Autodesk Inventor part; units mm, degrees
ref_plane "YZ Plane" through (0, 0, 0) normal (1, 0, 0) x (0, 1, 0)
ref_plane "XZ Plane" through (0, 0, 0) normal (0, 1, 0) x (-1, 0, 0)
ref_plane "XY Plane" through (0, 0, 0) normal (0, 0, 1) x (1, 0, 0)
sketch "Sketch1" plane through (0, 0, 0) normal (0, 1, 0) x (-1, 0, 0)
  line L0 (-7.5, 15) -> (7.5, 15)
  line L1 (7.5, 15) -> (7.5, -15)
  line L2 (7.5, -15) -> (-7.5, -15)
  line L3 (-7.5, -15) -> (-7.5, 15)
  line L4 (-7.5, 15) -> (7.5, -15) construction
  line L5 (7.5, 15) -> (-7.5, -15) construction
  point P0 (0, 0)
  dimension "d0" = 15
  dimension "d1" = 30
extrude "Extrusion1" add sketch "Sketch1" along normal blind 4
chamfer "Chamfer1" distance 2.5 distance2 1 1 edges at (7.5, 2, -15) measured on face at (7.5, 1.3333, 5)
chamfer "Chamfer2" distance 1 distance2 2.5 1 edges at (-7.5, 2, -15) measured on face at (1.8333, 2.6667, -15)
sketch "Sketch3" plane through (0, 0, 0) normal (0, -1, 0) x (1, 0, 0)
  line L0 (0, 0) -> (4, 0)
  line L1 (0, 0) -> (-4, 0)
  dimension "d14" = 4
  dimension "d15" = 4
hole "Hole1" at (4, 0, 0) at (-4, 0, 0) direction (0, 1, 0) diameter 2.1565 end through all
sketch "Sketch4" plane through (0, 0, 0) normal (0, -1, 0) x (1, 0, 0)
  line L0 (7.5, 15) -> (7.5, -12.5)
  line L1 (7.5, -12.5) -> (7.5, -7.5)
  line L2 (7.5, -7.5) -> (2.5, -7.5)
  line L3 (2.5, -7.5) -> (2.5, -5.5)
  line L4 (2.5, -5.5) -> (-2.5, -5.5)
  line L5 (-2.5, -5.5) -> (-2.5, -7.5)
  line L6 (-2.5, -7.5) -> (-7.5679, -7.5)
  line L7 (-7.5679, -7.5) -> (-7.5679, -12.5)
  line L8 (6.5, -15) -> (-6.5, -15)
  line L9 (-7.5679, -12.5) -> (-6.5, -15)
  line L10 (7.5, -12.5) -> (6.5, -15)
  line L11 (-6.5, -15) -> (6.5, -15)
  line L12 (6.5, -15) -> (7.5, -12.5)
  point P0 (0, 0)
  dimension "d23" = 5
  dimension "d24" = 5
  dimension "d25" = 2
  dimension "d26" = 5
split body "Split1" sketch "Sketch4" result one side removed curves L2 L3 L4 L5 L6 L7 L9 L11 L12 L1 removed pieces at (1.1663, 0.5, 10.3182)
sketch "Sketch5" plane through (-7.5, 0, -12.5) normal (-1, 0, 0) x (0, 0, 1)
  line L0 (0, 0) -> (0, 4)
  line L1 (-2.5, 4) -> (-2.5, 0)
  line L2 (0, 0) -> (-2.5, 0)
  line L3 (-2.5, 0) -> (-2.5, 4)
  line L4 (-2.5, 4) -> (0, 4)
  line L5 (0, 4) -> (0, 0)
  point P0 (12.5, 0)
extrude "Extrusion3" cut sketch "Sketch5" against normal blind 2
sketch "Sketch6" plane through (7.5, 0, -12.5) normal (1, 0, 0) x (0, 0, -1)
  line L0 (0, 4) -> (0, 0)
  line L1 (2.5, 0) -> (2.5, 4)
  line L2 (0, 4) -> (2.5, 4)
  line L3 (2.5, 4) -> (2.5, 0)
  line L4 (2.5, 0) -> (0, 0)
  line L5 (0, 0) -> (0, 4)
  point P0 (-12.5, 0)
extrude "Extrusion4" cut sketch "Sketch6" against normal blind 2
hole "Hole2" at (-7.5, 2, -10) direction (1, 0, 0) diameter 2.5 depth 7.5
sketch "Sketch7" plane through (-7.5, 0, -12.5) normal (0, 0, -1) x (-1, 0, 0)
  line L0 (0, 0) -> (0, 4)
  line L1 (-2, 4) -> (0, 4)
  line L2 (-2, 4) -> (-2, 0)
  line L3 (0, 0) -> (-2, 0)
  point P0 (-7.5, 0)
extrude "Extrusion5" cut sketch "Sketch7" against normal blind 0.5
sketch "Sketch8" plane through (7.5, 0, -12.5) normal (0, 0, -1) x (-1, 0, 0)
  line L0 (2, 0) -> (0, 0)
  line L1 (0, 4) -> (0, 0)
  line L2 (2, 0) -> (0, 0)
  line L3 (2, 0) -> (2, 4)
  line L4 (0, 4) -> (2, 4)
  point P0 (7.5, 0)
extrude "Extrusion6" cut sketch "Sketch8" against normal blind 0.5
sketch "Sketch9" plane through (-5.5, 0, -12.5) normal (-1, 0, 0) x (0, 0, 1)
  line L0 (-2.5, 0) -> (-2.5, 4)
  line L1 (-2.5, 2) -> (-1.013, 2)
  point P0 (12.5, 0)
  dimension "d44" = 1.487
hole "Hole3" [suppressed]
sketch "Sketch10" plane through (5.5, 0, -12.5) normal (1, 0, 0) x (0, 0, -1)
  circle A0 centre (1.013, 2) radius 0.5953
  point P0 (-12.5, 0)
hole "Hole4" [suppressed]
sketch "Sketch11" plane through (-5.5, 0, -15) normal (0, 0, -1) x (-1, 0, 0)
  line L0 (-11, 4) -> (-11, 0)
  line L1 (-11, 0) -> (0, 0)
  line L2 (-11, 4) -> (0, 4)
  line L3 (0, 4) -> (0, 0)
  line L4 (0, 0) -> (-11, 0)
  line L5 (-11, 0) -> (-11, 4)
  point P0 (-5.5, 0)
extrude "Extrusion7" cut sketch "Sketch11" against normal blind 0.5
sketch "Sketch12" plane through (0, 2, -10) normal (-1, 0, 0) x (0, 0, 1)
  circle A0 centre (-0.55, 0) radius 0.15
  circle A1 centre (0.55, 0) radius 0.15
  point P0 (10, -2)
  dimension "d63" = 0.3
  dimension "d64" = 0.3
extrude "Extrusion8" add sketch "Sketch12" along normal blind 25
sketch "Sketch13" plane through (-25, 2, -10.55) normal (-1, 0, 0) x (0, 0, 1)
  circle A0 centre (0, 0) radius 0.15
  circle A1 centre (0, 0) radius 0.075
  circle A2 centre (1.1, 0) radius 0.15
  circle A3 centre (1.1, 0) radius 0.075
  circle A4 centre (0, 0) radius 0.15
  circle A5 centre (1.1, 0) radius 0.15
  point P0 (10.55, -2)
  dimension "d67" = 0.15
  dimension "d68" = 0.15
extrude "Extrusion9" cut sketch "Sketch13" against normal blind 5
properties part number "AlN_thermal_contact" material "Copper"
Verification items for the finished model (mm, model axes). A direction names the side the tool comes from. Give positions to 0.01 mm unless a question says otherwise; leave off trailing zeros. Write each loop counter-clockwise with the first axis right and the second up, starting at its lowest first coordinate (ties: lowest second). Pieces come first, ordered by that corner, then holes.
(1) Material ranges on line 1 (Y direction, x = -5.75, z = -10); line 2 (X direction, y = 0.5, z = -7.75); line 3 (X direction, y = 2.8, z = -9.75), recorded low to high.
(2) Cross-section at D-D (z = -6.5). Enter the section's corners in (x, y).
(3) Mould release check, pull along Z, two halves, no side actions. Record for faces 6 (the face through (0, 2, -10)), 7 (the face through (-6, 2, -12)), 8 (the face through (-5, 2, -7.5)), 9 (the face through (2.5, 2, -7)): +Z half, -Z half, draft (parallel to the pull), parting line (faces both ways), or undercut.
(4) Gauge pin test, flat ends, axial feed: pin 1 (0.6 mm diameter, centred on x = -7, y = 1, fed in from -Z); pin 2 (0.8 mm diameter, centred on y = 2.5, z = -13, fed in from +X); pin 3 (1.2 mm diameter, centred on y = 1.5, z = -13, fed in from -X). Record the tip position at first contact, or that the pin passes through.
(5) Cross-section at C-C (y = 1.3). Enter the section's corners in (x, z), plus the area to 3 significant figures.
(6) Access from +Z, -Z, +X, -X, +Y, -Y to the whole of each face (thin tool, end or side, straight path). Record for faces 1 (the face through (-5.5, 2, -13)), 2 (the face through (-2.5, 2, -6)), 3 (the face through (-3.7, 1.95, -11.25)), 4 (the face through (5, 2, -7.5)), 5 (the face through (7, 2, -12)).
(7) Cross-section at B-B (x = -15). Enter the section's corners in (y, z), plus the area to 3 significant figures.
(8) Cross-section at A-A (z = -10). Enter the section's corners in (x, y).
Worked out:
1. line 1: y = 0 to 0.75, 3.25 to 4
1. line 2: x = -7.5 to 7.5
1. line 3: x = 0 to 7.5
2. outline: (-2.5, 0) - (2.5, 0) - (2.5, 4) - (-2.5, 4) - close
3. face 6: undercut
3. face 7: -Z half
3. face 8: +Z half
3. face 9: draft
4. pin 1: stops at z = -12
4. pin 2: stops at x = 5.5
4. pin 3: stops at x = -5.5
5. outline: (-7.5, -12) - (-5.5, -12) - (-5.5, -14.5) - (5.5, -14.5) - (5.5, -12) - (7.5, -12) - (7.5, -7.5) - (2.5, -7.5) - (2.5, -5.5) - (-2.5, -5.5) - (-2.5, -7.5) - (-7.5, -7.5) - (-7.5, -8.96) - (0, -8.96) - (0, -11.04) - (-7.5, -11.04) - close
5. area: 89.5 mm2
6. face 1: -Z, -X, +Y, -Y
6. face 2: +Z, -X, +Y, -Y
6. face 3: -X
6. face 4: +Z, +X, +Y, -Y
6. face 5: -Z, +X, +Y, -Y
7. outline: circle Ø0.3 at (2, -10.55); circle Ø0.3 at (2, -9.45)
7. area: 0.141 mm2
8. outline: (-7.5, 0) - (7.5, 0) - (7.5, 4) - (-7.5, 4) - (-7.5, 3.25) - (0, 3.25) - (0, 0.75) - (-7.5, 0.75) - close
